```python
from build123d import *

# Parameters (mm, degrees)
ESQUISSE1_W             = 330
ESQUISSE1_H             = 54
BOSS_EXTRU_1_DEPTH      = 6
ESQUISSE2_W             = 6
ESQUISSE2_H             = 14
ENL_V_MAT_EXTRU_1_DEPTH = 335.442820225
ESQUISSE4_W             = 318
ESQUISSE4_H             = 8.870374263
ENL_V_MAT_EXTRU_2_DEPTH = 1


with BuildPart() as part:
    # Esquisse1 → Boss.-Extru.1 (new body)
    with BuildSketch(Plane.XY):
        with Locations((-165, 27)):
            Rectangle(ESQUISSE1_W, ESQUISSE1_H)
    extrude(amount=BOSS_EXTRU_1_DEPTH)

    # Esquisse2 → Enlèv. mat.-Extru.1 (cut, through all)
    with BuildSketch(Plane.XY.offset(6)):
        Polygon((-330, 0), (-175, 0), (-175, 6), (-324, 6), (-324, 20), (-330, 20), align=None)
        with Locations((-327, 47)):
            Rectangle(ESQUISSE2_W, ESQUISSE2_H)
        Polygon((-155, 0), (0, 0), (0, 20), (-6, 20), (-6, 6), (-155, 6), align=None)
        with Locations((-3, 47)):
            Rectangle(ESQUISSE2_W, ESQUISSE2_H)
    extrude(amount=-ENL_V_MAT_EXTRU_1_DEPTH, mode=Mode.SUBTRACT)

    # Esquisse4 → Enlèv. mat.-Extru.2 (cut)
    with BuildSketch(Plane(origin=(0, 0, 0), x_dir=(-1, 0, 0), z_dir=(0, 0, -1))):
        with Locations((165, 49.564812868)):
            Rectangle(ESQUISSE4_W, ESQUISSE4_H)
    extrude(amount=-ENL_V_MAT_EXTRU_2_DEPTH, mode=Mode.SUBTRACT)


solid = part.part
```
Work out the finished part from the listing and answer in its coordinate system (mm). A direction names the side the tool comes from. Coordinates: 2 decimals unless noted, no trailing zeros. Loops run counter-clockwise (first coordinate to the right, second up) from the corner with the lowest first, then second, coordinate; pieces in that order, holes last.
1) Section B-B (x = -193.5) is taken. Give the vertices of the cut face in (y, z), plus the area to 3 significant figures.
Results:
outline: (6, 0) - (45.13, 0) - (45.13, 1) - (54, 1) - (54, 6) - (6, 6) - close
area: 279 mm2
2) Section A-A (z = 2.25) is taken. Give the vertices of the cut face in (x, y).
Results:
outline: (-330, 20) - (-324, 20) - (-324, 6) - (-175, 6) - (-175, 0) - (-155, 0) - (-155, 6) - (-6, 6) - (-6, 20) - (0, 20) - (0, 40) - (-6, 40) - (-6, 54) - (-324, 54) - (-324, 40) - (-330, 40) - close
3) Flat-ended cylindrical pins translate along their axes: pin 1 (1.5 mm diameter, centred on y = 7, z = 4.5, fed in from -X); pin 2 (1.8 mm diameter, centred on y = 12, z = 3, fed in from +X); pin 3 (0.8 mm diameter, centred on x = -242, z = 0.5, fed in from +Y). Find the tip coordinate at first contact, or state that the pin passes through.
Results:
pin 1: stops at x = -324
pin 2: stops at x = -6
pin 3: stops at y = 45.13
4) For faces 1 (the flat face through (-3, 40, 3)), 2 (the flat face through (-155, 3, 3)), 3 (the flat face through (-324, 13, 3)), 4 (the flat face through (-324, 47, 3)), 5 (the flat face through (-163, 50, 1)), determine the directions among +Z, -Z, +X, -X, +Y, -Y from which every point of the face is accessible in a straight line to the end or side of a thin tool.
Results:
face 1: +Z, -Z, +X, +Y
face 2: +Z, -Z, +X, -Y
face 3: +Z, -Z, -X, -Y
face 4: +Z, -Z, -X, +Y
face 5: -Z, +X, -X, +Y
5) Consider probe 1 along Y at (x, z) = (-194, 2.5); probe 2 along Y at (x, z) = (-65, 0.8); probe 3 along Z at (x, y) = (-314.5, 45.5). Determine where each line is inside the solid, lowest interval first.
Results:
probe 1: y = 6 to 54
probe 2: y = 6 to 45.13
probe 3: z = 1 to 6
6) Section C-C (y = 51) is taken. Give the vertices of the cut face in (x, z), plus the area to 3 significant figures.
Results:
outline: (-324, 1) - (-6, 1) - (-6, 6) - (-324, 6) - close
area: 1,590 mm2
7) Section D-D (y = 17) is taken. Give the vertices of the cut face in (x, z), plus the area to 3 significant figures.
Results:
outline: (-324, 0) - (-6, 0) - (-6, 6) - (-324, 6) - close
area: 1,910 mm2
